```python
from build123d import *

# Parameters (mm, degrees)
SKETCH3_W           = 100
SKETCH3_H           = 50
BOSS_EXTRUDE1_DEPTH = 35
SKETCH4_W           = 25
SKETCH4_H           = 40
CUT_EXTRUDE2_DEPTH  = 100
SKETCH5_R           = 4.002277078
CUT_EXTRUDE4_DEPTH  = 5
FILLET2_R           = 5
FILLET3_R           = 5
FILLET4_R           = 5
FILLET5_R           = 5
SCALE1_SCALE        = 0.15


with BuildPart() as part:
    # Sketch3 → Boss-Extrude1 (new body)
    with BuildSketch(Plane.XY):
        with Locations((2.343116294, 2.356397797)):
            Rectangle(SKETCH3_W, SKETCH3_H)
    extrude(amount=BOSS_EXTRUDE1_DEPTH)

    # Sketch4 → Cut-Extrude2 (cut)
    with BuildSketch(Plane.ZY.offset(47.656883706)):
        with Locations((17.5, 2.356397797)):
            Rectangle(SKETCH4_W, SKETCH4_H)
    extrude(amount=-CUT_EXTRUDE2_DEPTH, mode=Mode.SUBTRACT)

    # Sketch5 → Cut-Extrude4 (cut)
    with BuildSketch(Plane.XY.offset(35)):
        with Locations((-5.550407573, 12.303618629)):
            Circle(SKETCH5_R)
        with Locations(Location((10.236640162, 12.303618629, 0), (0, 0, 180))):
            Circle(SKETCH5_R)
    extrude(amount=-CUT_EXTRUDE4_DEPTH, mode=Mode.SUBTRACT)

    # Fillet2
    fillet2_edges = [part.edges().sort_by_distance(p)[0] for p in [
        (2.343116294, 22.356397797, 5),
    ]]
    fillet(fillet2_edges, radius=FILLET2_R)

    # Fillet3
    fillet3_edges = [part.edges().sort_by_distance(p)[0] for p in [
        (2.343116294, 22.356397797, 30),
    ]]
    fillet(fillet3_edges, radius=FILLET3_R)

    # Fillet4
    fillet4_edges = [part.edges().sort_by_distance(p)[0] for p in [
        (2.343116294, -17.643602203, 5),
    ]]
    fillet(fillet4_edges, radius=FILLET4_R)

    # Fillet5
    fillet5_edges = [part.edges().sort_by_distance(p)[0] for p in [
        (2.343116294, -17.643602203, 30),
    ]]
    fillet(fillet5_edges, radius=FILLET5_R)


with BuildPart() as part_1:
    # Scale1: scaled about (2.343116294, 2.291085551, 17.401511818)
    add(part.part.scale(SCALE1_SCALE).moved(Location((1.99164885, 1.947422718, 14.791285045))))


solid = part_1.part
```
Here's how the part is built. I have some questions about the finished solid (model axes, mm). A direction names the side the tool comes from. Round coordinates to 2 decimals unless told otherwise and drop trailing zeros. Order: outer loops, then holes, each group sorted by start corner. A loop starts at its lowest first (then second) coordinate and runs counter-clockwise, first axis right, second up. Notation, with made-up numbers: M -28,-15 L 0,-15 A11 cw 0,6 Z; hole C 64.5,-5 d3. An arc over 180 degrees is marked long. Answer in a Markdown table with one row per item.
Item 1: I'm going to push a flat-ended pin straight in: pin 1 (1.5 mm diameter, centred on y = 0.5, z = 19, fed in from -X). Where does the tip first touch, or does it pass through?
A:
| item | result |
|---|---|
| pin 1 | stops at x = -5.16 |
Item 2: Imagine slicing it at A-A, the plane z = 17.35. Write out the boundary of the cut face in (x, y), and give its area (3 significant figures).
A:
| item | result |
|---|---|
| outline | M -5.16,-1.45 L 9.84,-1.45 L 9.84,-0.7 L -5.16,-0.7 Z; M -5.16,5.3 L 9.84,5.3 L 9.84,6.05 L -5.16,6.05 Z |
| area | 22.5 mm2 |
Item 3: Imagine slicing it at D-D, the plane y = 4. Write out the boundary of the cut face in (x, z), and give its area (3 significant figures).
A:
| item | result |
|---|---|
| outline | M -5.16,14.79 L 9.84,14.79 L 9.84,15.54 L -5.16,15.54 Z; M -5.16,19.29 L 0.6,19.29 L 0.6,20.04 L -5.16,20.04 Z; M 1.72,19.29 L 2.96,19.29 L 2.96,20.04 L 1.72,20.04 Z; M 4.09,19.29 L 9.84,19.29 L 9.84,20.04 L 4.09,20.04 Z |
| area | 20.8 mm2 |
Item 4: Imagine slicing it at C-C, the plane y = 1. Write out the boundary of the cut face in (x, z).
A:
| item | result |
|---|---|
| outline | M -5.16,14.79 L 9.84,14.79 L 9.84,15.54 L -5.16,15.54 Z; M -5.16,19.29 L 9.84,19.29 L 9.84,20.04 L -5.16,20.04 Z |
Item 5: If I drill on L1, parallel to Y at x = -2, z = 16.7; L2, parallel to Z at x = 1.25, y = 1.5; L3, parallel to Y at x = 3.5, z = 15.8, over which ranges is the centre line in solid material (lowest first)? Write a range as from..to.
A:
| item | result |
|---|---|
| L1 | y = -1.45..-0.7, 5.3..6.05 |
| L2 | z = 14.79..15.54, 19.29..20.04 |
| L3 | y = -1.45..-0.52, 5.12..6.05 |
Item 6: For faces 5 (the face through (2, 2, 14.791)), 6 (the face through (2, 2, 15.541)), 7 (the face through (1.029, 3.207, 19.672)), which set-ups out of +Z, -Z, +X, -X, +Y, -Y let a thin tool reach every point of the face, with its end or its side?
A:
| item | result |
|---|---|
| face 5 | -Z, +X, -X, +Y, -Y |
| face 6 | +X, -X |
| face 7 | +Z |
Item 7: Imagine slicing it at B-B, the plane x = -4. Write out the boundary of the cut face in (y, z), and give its area (3 significant figures).
A:
| item | result |
|---|---|
| outline | M -1.45,14.79 L 6.05,14.79 L 6.05,20.04 L -1.45,20.04 Z; hole M -0.7,16.29 A0.75 ccw 0.05,15.54 L 4.55,15.54 A0.75 ccw 5.3,16.29 L 5.3,18.54 A0.75 ccw 4.55,19.29 L 0.05,19.29 A0.75 ccw -0.7,18.54 Z |
| area | 17.4 mm2 |
Item 8: Thinking about a two-plate mould opening in Y: for faces 1 (the face through (2, 2, 20.041)), 2 (the face through (4, 4.16, 19.67)), 3 (the face through (2, -0.699, 17)), 4 (the face through (2, -1.449, 17)), which applies, +Y half, -Y half, draft (parallel to the pull), parting line (faces both ways), or undercut?
A:
| item | result |
|---|---|
| face 1 | draft |
| face 2 | undercut |
| face 3 | undercut |
| face 4 | -Y half |
